Source: CAD feature listing. Evaluate the final solid. Frame: model axes, mm. A direction names the side the tool comes from. Coordinates: 2 decimals unless noted, no trailing zeros. Order: outer loops, then holes, each group sorted by start corner. A loop starts at its lowest first (then second) coordinate and runs counter-clockwise, first axis right, second up. Notation, with made-up numbers: (28, 5.5) -> (50, 5.5) arc R17 cw to (50, 24.5) -> close; hole circle Ø5 at (-39, 80). An arc over 180 degrees is marked (long way). Put each result on its own line as item: value.
from build123d import *

# Parameters (mm, degrees)
SKETCH2_W           = 48.26
SKETCH2_H           = 7.62
BOSS_EXTRUDE1_DEPTH = 2.54
SKETCH3_W           = 5.026957718
SKETCH3_H           = 15.24
BOSS_EXTRUDE2_DEPTH = 2.54
SKETCH4_R           = 1.030507416
CUT_EXTRUDE1_DEPTH  = 2.54
SKETCH5_W           = 7.62
SKETCH5_H           = 7.62
BOSS_EXTRUDE3_DEPTH = 2.54
SKETCH6_R           = 1.55
CUT_EXTRUDE2_DEPTH  = 2.54


with BuildPart() as part:
    # Sketch2 → Boss-Extrude1 (new body)
    with BuildSketch(Plane.XY):
        with Locations((24.13, 3.81)):
            Rectangle(SKETCH2_W, SKETCH2_H)
    extrude(amount=BOSS_EXTRUDE1_DEPTH)

    # Sketch3 → Boss-Extrude2 (add)
    with BuildSketch(Plane.XY):
        with Locations((-2.513478859, 7.62)):
            Rectangle(SKETCH3_W, SKETCH3_H)
    extrude(amount=BOSS_EXTRUDE2_DEPTH)

    # Sketch4 → Cut-Extrude1 (cut)
    with BuildSketch(Plane.XY.offset(2.54)):
        with Locations((-2.586282317, 12.7)):
            Circle(SKETCH4_R)
    extrude(amount=-CUT_EXTRUDE1_DEPTH, mode=Mode.SUBTRACT)

    # Sketch5 → Boss-Extrude3 (add)
    with BuildSketch(Plane.ZY.offset(-48.26)):
        with Locations((6.35, 3.81)):
            Rectangle(SKETCH5_W, SKETCH5_H)
    extrude(amount=BOSS_EXTRUDE3_DEPTH)

    # Sketch6 → Cut-Extrude2 (cut)
    with BuildSketch(Plane.ZY.offset(-45.72)):
        with Locations((6.35, 3.81)):
            Circle(SKETCH6_R)
    extrude(amount=-CUT_EXTRUDE2_DEPTH, mode=Mode.SUBTRACT)


solid = part.part
1. Cut plane C-C on z = 6.35. Output: boundary loops of the cut face in (x, y), plus the area to 3 significant figures.
Numbers:
outline: (45.72, 0) -> (48.26, 0) -> (48.26, 2.26) -> (45.72, 2.26) -> close; (45.72, 5.36) -> (48.26, 5.36) -> (48.26, 7.62) -> (45.72, 7.62) -> close
area: 11.5 mm2
2. Set-up query: faces 5 (the flat face through (45.72, 2, 6)), 6 (the flat face through (26, 7.62, 2)), 7 (the flat face through (48.26, 5, 5)). Return all of +Z, -Z, +X, -X, +Y, -Y with unobstructed straight access to the full face (end or side cutting, diameter ignored); none if empty.
Numbers:
face 5: +Z, -X, +Y, -Y
face 6: +Z, -Z, +X, +Y
face 7: +Z, -Z, +X, +Y, -Y
3. Pull-direction query (X, two-part tool) for faces 1 (the cylindrical face through (-2.111, 11.786, 1.288)), 2 (the flat face through (0, 11, 1)), 3 (the flat face through (-5.027, 8, 1)), 4 (the flat face through (47, 4, 10.16)); classes: pulls with the +X half, pulls with the -X half, needs draft (parallel to the pull), parting line crosses it, or undercut.
Numbers:
face 1: undercut
face 2: pulls with the +X half
face 3: pulls with the -X half
face 4: needs draft
4. Cut plane D-D on y = 12.7. Output: boundary loops of the cut face in (x, z).
Numbers:
outline: (-5.03, 0) -> (-3.62, 0) -> (-3.62, 2.54) -> (-5.03, 2.54) -> close; (-1.56, 0) -> (0, 0) -> (0, 2.54) -> (-1.56, 2.54) -> close
5. Ray query, line 1 along Y through (x, z) = (47.35, 6.35); line 2 along Z through (x, y) = (36.5, 2.5); line 3 along X through (y, z) = (2.25, 8.75). Return the intervals inside material, ascending.
Numbers:
line 1: y = 0 to 2.26, 5.36 to 7.62
line 2: z = 0 to 2.54
line 3: x = 45.72 to 48.26
6. Cut plane B-B on y = 3.81. Output: boundary loops of the cut face in (x, z), plus the area to 3 significant figures.
Numbers:
outline: (-5.03, 0) -> (48.26, 0) -> (48.26, 4.8) -> (45.72, 4.8) -> (45.72, 2.54) -> (-5.03, 2.54) -> close; (45.72, 7.9) -> (48.26, 7.9) -> (48.26, 10.16) -> (45.72, 10.16) -> close
area: 147 mm2
7. First-contact query: pin 1 (4 mm diameter, centred on y = 6.5, z = 5.5, fed in from -X); pin 2 (1.5 mm diameter, centred on x = 7.5, z = 4, fed in from +Y); pin 3 (5 mm diameter, centred on x = 17, z = 2.5, fed in from +Y); pin 4 (8 mm diameter, centred on x = 33, y = 9, fed in from +Z). Flat tips, straight axial feed; report the tip coordinate or a pass-through.
Numbers:
pin 1: stops at x = 45.72
pin 2: passes through
pin 3: stops at y = 7.62
pin 4: stops at z = 2.54
8. Cut plane A-A on z = 1.5. Output: boundary loops of the cut face in (x, y), plus the area to 3 significant figures.
Numbers:
outline: (-5.03, 0) -> (48.26, 0) -> (48.26, 7.62) -> (0, 7.62) -> (0, 15.24) -> (-5.03, 15.24) -> close; hole circle Ø2.06 at (-2.59, 12.7)
area: 441 mm2
